Build history of the part. All positions in model axes, mm. A direction names the side the tool comes from. Coordinates: 2 decimals unless noted, no trailing zeros. Order: outer loops, then holes, each group sorted by start corner. A loop starts at its lowest first (then second) coordinate and runs counter-clockwise, first axis right, second up. Notation, with made-up numbers: (-6.75, 65) - (4.25, 65) arc R20 ccw to (4.25, 83) - close; hole circle Ø6 at (-12.75, -33). An arc over 180 degrees is marked (long way). Return JSON: item names as keys, results as strings.
Autodesk Inventor part; units mm, degrees
ref_plane "YZ Plane" through (0, 0, 0) normal (1, 0, 0) x (0, 1, 0)
ref_plane "XZ Plane" through (0, 0, 0) normal (0, 1, 0) x (-1, 0, 0)
ref_plane "XY Plane" through (0, 0, 0) normal (0, 0, 1) x (1, 0, 0)
sketch "スケッチ1" plane through (0, 0, 0) normal (0, 0, 1) x (1, 0, 0)
  line L0 (0, 2.8868) -> (2.5, 1.4434)
  line L1 (2.5, 1.4434) -> (2.5, -1.4434)
  line L2 (2.5, -1.4434) -> (0, -2.8868)
  line L3 (0, -2.8868) -> (-2.5, -1.4434)
  line L4 (-2.5, -1.4434) -> (-2.5, 1.4434)
  line L5 (-2.5, 1.4434) -> (0, 2.8868)
  point P0 (0, 0)
  point P1 (0, 0)
  dimension "d0" = 5
extrude "押し出し1" add sketch "スケッチ1" along normal blind 20
sketch "スケッチ2" plane through (0, 0, 20) normal (0, 0, 1) x (1, 0, 0)
  circle A0 centre (0, 0) radius 1.3
  dimension "d3" = 2.6
extrude "押し出し2" add sketch "スケッチ2" along normal blind 5
thread "ねじ1"
sketch "スケッチ3" plane through (0, 0, 0) normal (0, 0, -1) x (-1, 0, 0)
  point P0 (0, 0)
hole "穴1" at (0, 0, 0) direction (0, 0, 1) diameter 2.113 depth 6 tip angle 118
properties part number "ジュラコンスペーサー（六角）_BS-2620E" material "アセタール樹脂、白"
1. Cut at B-B on y = 1.95. Give the cut face in (x, z).
Check values:
{"outline": "(-1.62, 0) - (1.62, 0) - (1.62, 20) - (-1.62, 20) - close"}
2. Mould opens along X. For faces 3 (the flat face through (-2.5, 0, 10)), 4 (the conical face through (-0.112, -0.146, 6.525)), 5 (the cylindrical face through (1.03, -0.23, 3.04)), 6 (the flat face through (2.5, 0, 10)) say: pulls with the +X half, pulls with the -X half, needs draft (parallel to the pull), parting line crosses it, or undercut.
Check values:
{"face 3": "pulls with the -X half", "face 4": "undercut", "face 5": "undercut", "face 6": "pulls with the +X half"}
3. Cut at D-D on z = 21.5. Give the cut face in (x, y), plus the area to 3 significant figures.
Check values:
{"outline": "circle Ø2.6 at (0, 0)", "area": "5.31 mm²"}
4. Tool access for faces 1 (the cylindrical face through (-0.17, -1.29, 22.46)), 2 (the flat face through (1.267, -2.155, 9.86)): list every direction of +Z, -Z, +X, -X, +Y, -Y with a clear straight run to the whole face (end or side of a thin tool).
Check values:
{"face 1": "+Z", "face 2": "+Z, -Z, +X, -Y"}
5. Drop flat-ended pins along their axis: pin 1 (1.5 mm diameter, centred on x = 1, y = -1.5, fed in from +Z); pin 2 (1.3 mm diameter, centred on x = 0, y = 0, fed in from -Z). Give the stop position or say it passes through.
Check values:
{"pin 1": "z = 25", "pin 2": "z = 6.24"}
6. Cut at A-A on z = 10. Give the cut face in (x, y).
Check values:
{"outline": "(-2.5, -1.44) - (0, -2.89) - (2.5, -1.44) - (2.5, 1.44) - (0, 2.89) - (-2.5, 1.44) - close"}
7. Cut at C-C on x = 1.8. Give the cut face in (y, z), plus the area to 3 significant figures.
Check values:
{"outline": "(-1.85, 0) - (1.85, 0) - (1.85, 20) - (-1.85, 20) - close", "area": "73.9 mm²"}
8. Probe L1, parallel to X at y = 0, z = 3.65; L2, parallel to Z at x = 1.6, y = 0.8; L3, parallel to X at y = 0.9, z = 2.5. List the from-to ranges inside material, lowest first.
Check values:
{"L1": "-2.5 to -1.06, 1.06 to 2.5", "L2": "0 to 20", "L3": "-2.5 to -0.55, 0.55 to 2.5"}
